Verification items for the finished model (mm, model axes). A direction names the side the tool comes from. Round coordinates to 2 decimals unless told otherwise and drop trailing zeros. Write each loop counter-clockwise with the first axis right and the second up, starting at its lowest first coordinate (ties: lowest second). Pieces come first, ordered by that corner, then holes. Notation, with made-up numbers: (-27.5, -19) - (17.5, -19) arc R14 cw to (17.5, -5) - close; hole circle Ø11 at (59, -25). An arc over 180 degrees is marked (long way). Answer as a JSON object with one key per item and string values. Group by question number.
1) Mould release check, pull along X, two halves, no side actions. Record for faces 4 (the cylindrical face through (6.77, -48.136, -1.634)), 5 (the cylindrical face through (-15.497, -42.885, -3.441)), 6 (the flat face through (0, -57.15, 0)): +X half, -X half, draft (parallel to the pull), parting line (faces both ways), or undercut.
2) Section check A-A (x = 0). State how many separate pieces and enclosed holes the cut face has, then the cut area to 3 significant figures.
3) Section check C-C (x = -22.86). Enter the section's corners in (y, z).
4) Set-up check for faces 1 (the conical face through (3.86, -47.47, 12.26)), 2 (the flat face through (-14, -6.35, 14)), 3 (the cylindrical face through (-30.995, -3.219, -6.883)): record each of +Z, -Z, +X, -X, +Y, -Y from which the full face is reachable in a straight line by a thin tool's end or side.
5) Section check B-B (z = -22.86). Enter the section's corners in (x, y), then the cut area to 3 significant figures.
6) Go/stop test with flat-tipped pins: pin 1 Ø6 at (x, y) = (7.5, -35) entering from -Z; pin 2 Ø4.5 at (x, z) = (-22.86, 0) entering from +Y; pin 3 Ø10 at (y, z) = (-10, -12.5) entering from -X; pin 4 Ø8 at (x, z) = (-22, 18.5) entering from -Y. Record where each tip stops, or that it passes through.
7) Thickness scan on line 1 (X direction, y = -50.25, z = 0); line 2 (X direction, y = -1, z = 0); line 3 (Y direction, x = 11.5, z = -7.5). Record the ranges inside material, lowest first.
```python
from build123d import *

# Parameters (mm, degrees)
F3_D           = 3.302
F3_CSINK_D     = 5.08
F3_CSINK_ANGLE = 90
F5_D           = 3.683
F5_DEPTH       = 17.78
F5_TIP         = 1.1064848299
F6_R           = 5.08


with BuildPart() as f1:
    # F0 (on Right) → F1 (revolve)
    with BuildSketch(Plane.YZ):
        Polygon((-57.15, 0), (0, 0), (0, 31.75), (-6.35, 31.75), (-6.35, 12.7), (-38.1, 12.7), (-41.275, 15.875), (-44.45, 15.875), (-47.625, 12.7), (-50.8, 12.7), (-53.975, 15.875), (-57.15, 15.875), align=None)
    revolve(axis=Axis((0, -28.575, 0), (0, 1, 0)))

    # F3 (through all)
    with Locations(Plane.XZ.offset(6.35)):
        with Locations((0, 22.86), (22.86, 0), (0, -22.86), (-22.86, 0)):
            CounterSinkHole(F3_D / 2, F3_CSINK_D / 2, counter_sink_angle=F3_CSINK_ANGLE)

    # F5
    with Locations(Plane.XZ.offset(57.15)):
        with Locations((-7.62, 0), (7.62, 0)):
            Hole(F5_D / 2, depth=F5_DEPTH)
            with Locations((0, 0, -(F5_DEPTH + F5_TIP / 2))):  # 118° drill point
                Cone(0, F5_D / 2, F5_TIP, mode=Mode.SUBTRACT)

    # F6
    f6_edges = [f1.edges().sort_by_distance(p)[0] for p in [
        (0, -6.35, -12.7),
    ]]
    fillet(f6_edges, radius=F6_R)


solid = f1.part
```
Returned:
{
 "1": {"face 4": "undercut", "face 5": "parting line", "face 6": "draft"},
 "2": {"separate pieces": "3", "enclosed holes": "0", "area": "1,730 mm2"},
 "3": {"outline": "(-6.35, -22.03) - (0, -22.03) - (0, -1.65) - (-5.46, -1.65) - (-6.35, -2.54) - close; (-6.35, 2.54) - (-5.46, 1.65) - (0, 1.65) - (0, 22.03) - (-6.35, 22.03) - close"},
 "4": {"face 1": "none", "face 2": "-Y", "face 3": "+Y, -Y"},
 "5": {"outline": "(-22.03, -6.35) - (-2.54, -6.35) - (-1.65, -5.46) - (-1.65, 0) - (-22.03, 0) - close; (1.65, -5.46) - (2.54, -6.35) - (22.03, -6.35) - (22.03, 0) - (1.65, 0) - close", "area": "258 mm2"},
 "6": {"pin 1": "z = -11.88", "pin 2": "y = 0", "pin 3": "x = -30.42", "pin 4": "y = -6.35"},
 "7": {"line 1": "-12.7 to -9.46, -5.78 to 5.78, 9.46 to 12.7", "line 2": "-31.75 to -24.51, -21.21 to 21.21, 24.51 to 31.75", "line 3": "-57.15 to -51.83, -46.6 to -39.13, -8.36 to 0"}
}
